from build123d import *

# Parameters (mm, degrees)
SKETCH1_R           = 26.948722821
BOSS_EXTRUDE2_DEPTH = 72


with BuildPart() as part:
    # Sketch1 → Boss-Extrude2 (new body)
    with BuildSketch(Plane.XY):
        with BuildLine():
            Line((-9.649968123, 42.875568313), (-3.270074231, 56.514068549))
            Line((-3.270074231, 56.514068549), (3.270074231, 56.514068549))
            Line((3.270074231, 56.514068549), (9.649968123, 42.875568313))
            ThreePointArc((9.649968123, 42.875568313), (12.381612983, 42.167901333), (15.062212526, 41.28638997))
            Line((15.062212526, 41.28638997), (27.802850719, 49.310595427))
            Line((27.802850719, 49.310595427), (33.304773717, 45.774724216))
            Line((33.304773717, 45.774724216), (31.298352077, 30.852056661))
            ThreePointArc((31.298352077, 30.852056661), (33.213764311, 28.779890604), (34.992247123, 26.589074527))
            Line((34.992247123, 26.589074527), (50.048567011, 26.451356669))
            Line((50.048567011, 26.451356669), (52.765442869, 20.502228373))
            Line((52.765442869, 20.502228373), (43.00973039, 9.033235009))
            ThreePointArc((43.00973039, 9.033235009), (43.500780148, 6.254467957), (43.812490502, 3.449915791))
            Line((43.812490502, 3.449915791), (56.404216903, -4.806000935))
            Line((56.404216903, -4.806000935), (55.473456732, -11.279580116))
            Line((55.473456732, -11.279580116), (41.065823196, -15.653574932))
            ThreePointArc((41.065823196, -15.653574932), (39.97660565, -18.256704074), (38.72257771, -20.784566832))
            Line((38.72257771, -20.784566832), (44.851926462, -34.5374872))
            Line((44.851926462, -34.5374872), (40.56904004, -39.480201616))
            Line((40.56904004, -39.480201616), (26.083807295, -35.370485435))
            ThreePointArc((26.083807295, -35.370485435), (23.760141319, -36.971501558), (21.338520096, -38.420096343))
            Line((21.338520096, -38.420096343), (19.059466278, -53.303565309))
            Line((19.059466278, -53.303565309), (12.784239782, -55.146138057))
            Line((12.784239782, -55.146138057), (2.820366877, -43.857516729))
            ThreePointArc((2.820366877, -43.857516729), (0, -43.948108525), (-2.820366877, -43.857516729))
            Line((-2.820366877, -43.857516729), (-12.784239782, -55.146138057))
            Line((-12.784239782, -55.146138057), (-19.059466278, -53.303565309))
            Line((-19.059466278, -53.303565309), (-21.338520096, -38.420096343))
            ThreePointArc((-21.338520096, -38.420096343), (-23.760141319, -36.971501558), (-26.083807295, -35.370485435))
            Line((-26.083807295, -35.370485435), (-40.56904004, -39.480201616))
            Line((-40.56904004, -39.480201616), (-44.851926462, -34.5374872))
            Line((-44.851926462, -34.5374872), (-38.72257771, -20.784566832))
            ThreePointArc((-38.72257771, -20.784566832), (-39.97660565, -18.256704074), (-41.065823196, -15.653574932))
            Line((-41.065823196, -15.653574932), (-55.473456732, -11.279580116))
            Line((-55.473456732, -11.279580116), (-56.404216903, -4.806000935))
            Line((-56.404216903, -4.806000935), (-43.812490502, 3.449915791))
            ThreePointArc((-43.812490502, 3.449915791), (-43.500780148, 6.254467957), (-43.00973039, 9.033235009))
            Line((-43.00973039, 9.033235009), (-52.765442869, 20.502228373))
            Line((-52.765442869, 20.502228373), (-50.048567011, 26.451356669))
            Line((-50.048567011, 26.451356669), (-34.992247123, 26.589074527))
            ThreePointArc((-34.992247123, 26.589074527), (-33.213764311, 28.779890604), (-31.298352077, 30.852056661))
            Line((-31.298352077, 30.852056661), (-33.304773718, 45.774724216))
            Line((-33.304773718, 45.774724216), (-27.802850719, 49.310595427))
            Line((-27.802850719, 49.310595427), (-15.062212526, 41.28638997))
            ThreePointArc((-15.062212526, 41.28638997), (-12.381612983, 42.167901333), (-9.649968123, 42.875568313))
        make_face()
        Circle(SKETCH1_R, mode=Mode.SUBTRACT)
    extrude(amount=BOSS_EXTRUDE2_DEPTH)


solid = part.part
Check sheet for the modelled part. Datum: model origin and axes. Units: mm. A direction names the side the tool comes from. Give positions to 0.01 mm unless a question says otherwise; leave off trailing zeros. Loops run counter-clockwise (first coordinate to the right, second up) from the corner with the lowest first, then second, coordinate; pieces in that order, holes last. Notation, with made-up numbers: M 8.25,59.25 L 13.25,59.25 A6 cw 13.25,69.25 Z; hole C -15.75,26 d8. An arc over 180 degrees is marked long. Return JSON: item names as keys, results as strings. Group by question number.
1. Cross-section at A-A on x = 0. Record the boundary of the cut face in (y, z), plus the area to 3 significant figures.
2. Cross-section at B-B on y = 0. Record the boundary of the cut face in (x, z), plus the area to 3 significant figures.
3. Tool access check on faces 4 (the cylindrical face through (33.19, 28.81, 35.5)), 5 (the flat face through (51.388, 23.518, 35.496)), 6 (the flat face through (-6.505, 49.599, 35.496)), 7 (the flat face through (-48.169, -13.497, 35.496)), 8 (the cylindrical face through (23.79, -36.95, 35.5)). Record the directions out of +Z, -Z, +X, -X, +Y, -Y that give a thin tool (end or side, any length) a straight path to the whole face; none if there is none.
4. Cross-section at C-C on y = 38. Record the boundary of the cut face in (x, z).
5. Go/stop test with flat-tipped pins: pin 1 (1.5 mm diameter, centred on x = -16.5, z = 29, fed in from +Y); pin 2 (12 mm diameter, centred on x = -24, z = 15, fed in from -Y); pin 3 (6 mm diameter, centred on y = 45, z = 52.5, fed in from +X). Record where each tip stops, or that it passes through.
6. Thickness scan on L1, parallel to Y at x = 0, z = 38; L2, parallel to X at y = 45, z = 4; L3, parallel to X at y = 25, z = 35. Record the ranges inside material, lowest first.
7. Mould release check, pull along X, two halves, no side actions. Record for faces 1 (the flat face through (21.34, 45.24, 35.5)), 2 (the flat face through (-15.878, -54.238, 35.496)), 3 (the flat face through (-24, 14, 72)): released by +X, released by -X, zero draft, split by the parting line, or undercut.
Return value:
{
 "1": {"outline": "M -43.95,0 L -26.95,0 L -26.95,72 L -43.95,72 Z; M 26.95,0 L 56.51,0 L 56.51,72 L 26.95,72 Z", "area": "3,350 mm^2"},
 "2": {"outline": "M -49.07,0 L -26.95,0 L -26.95,72 L -49.07,72 Z; M 26.95,0 L 49.07,0 L 49.07,72 L 26.95,72 Z", "area": "3,190 mm^2"},
 "3": {"face 4": "+Z, -Z, +X", "face 5": "+Z, -Z, +X, +Y", "face 6": "+Z, -Z, +Y", "face 7": "+Z, -Z, -X", "face 8": "+Z, -Z, -Y"},
 "4": {"outline": "M -32.26,0 L 32.26,0 L 32.26,72 L -32.26,72 Z"},
 "5": {"pin 1": "y = 42.66", "pin 2": "y = -53.61", "pin 3": "x = 33.3"},
 "6": {"L1": "-43.95 to -26.95, 26.95 to 56.51", "L2": "-33.2 to -20.96, -8.66 to 8.66, 20.96 to 33.2", "L3": "-50.71 to -10.06, 10.06 to 50.71"},
 "7": {"face 1": "undercut", "face 2": "released by -X", "face 3": "zero draft"}
}
